Could you check a few things on this model? Use its own coordinates, in mm. Face numbers are marked on the shaded views. A direction names the side the tool comes from. Give positions to 0.01 mm unless a question says otherwise; leave off trailing zeros. Write each loop counter-clockwise with the first axis right and the second up, starting at its lowest first coordinate (ties: lowest second). Pieces come first, ordered by that corner, then holes. Notation, with made-up numbers: M 88,79.5 L 118,79.5 A14 cw 118,97.5 Z; hole C 48.5,-31 d9. An arc over 180 degrees is marked long. Answer as CSV lines item,"result". Start each with the question number.
from build123d import *

# Parameters (mm, degrees)
SKETCH2_R           = 2
BOSS_EXTRUDE1_DEPTH = 11
SKETCH3_R           = 2
BOSS_EXTRUDE2_DEPTH = 39
EXTRUDE_THIN1_REACH = 198.85
CUT_EXTRUDE2_START  = -6
SKETCH5_R           = 3
SKETCH5_R_2         = 2
CUT_EXTRUDE2_DEPTH  = 6


with BuildPart() as part:
    # Sketch2 → Boss-Extrude1 (new body)
    with BuildSketch(Plane(origin=(0, 0, 0), x_dir=(1, 0, 0), z_dir=(0, 1, 0))):
        with BuildLine():
            Line((0, -150), (29.793839815, -175))
            Line((29.793839815, -175), (69, -175))
            ThreePointArc((69, -175), (73.242640687, -173.242640687), (75, -169))
            Line((75, -169), (75, -6))
            ThreePointArc((75, -6), (73.242640687, -1.757359313), (69, 0))
            Line((69, 0), (6, 0))
            ThreePointArc((6, 0), (1.757359313, -1.757359313), (0, -6))
            Line((0, -6), (0, -150))
        make_face()
        with Locations(Location((69, -169, 0), (0, 0, 270))):
            Circle(SKETCH2_R, mode=Mode.SUBTRACT)
        with Locations(Location((69, -6, 0), (0, 0, 270))):
            Circle(SKETCH2_R, mode=Mode.SUBTRACT)
        with Locations(Location((6, -6, 0), (0, 0, 270))):
            Circle(SKETCH2_R, mode=Mode.SUBTRACT)
        with Locations(Location((39, -75, 0), (0, 0, 270))):
            Circle(SKETCH2_R, mode=Mode.SUBTRACT)
    extrude(amount=BOSS_EXTRUDE1_DEPTH)

    # Sketch3 → Boss-Extrude2 (add)
    with BuildSketch(Plane(origin=(0, 11, 0), x_dir=(1, 0, 0), z_dir=(0, 1, 0))):
        with BuildLine():
            Line((39, -67.5), (15, -67.5))
            Line((15, -67.5), (15, -15))
            Line((15, -15), (75, -15))
            Line((75, -15), (75, -6))
            ThreePointArc((75, -6), (73.242640687, -1.757359313), (69, 0))
            Line((69, 0), (6, 0))
            ThreePointArc((6, 0), (1.757359313, -1.757359313), (0, -6))
            Line((0, -6), (0, -150))
            Line((0, -150), (29.793839815, -175))
            Line((29.793839815, -175), (69, -175))
            ThreePointArc((69, -175), (73.242640687, -173.242640687), (75, -169))
            Line((75, -169), (75, -160))
            Line((75, -160), (35.253393329, -160))
            Line((35.253393329, -160), (15, -143.005385128))
            Line((15, -143.005385128), (15, -82.5))
            Line((15, -82.5), (39, -82.5))
            ThreePointArc((39, -82.5), (46.5, -75), (39, -67.5))
        make_face()
        with Locations(Location((69, -169, 0), (0, 0, 270))):
            Circle(SKETCH3_R, mode=Mode.SUBTRACT)
        with Locations(Location((6, -6, 0), (0, 0, 270))):
            Circle(SKETCH3_R, mode=Mode.SUBTRACT)
        with Locations(Location((39, -75, 0), (0, 0, 270))):
            Circle(SKETCH3_R, mode=Mode.SUBTRACT)
        with Locations(Location((69, -6, 0), (0, 0, 270))):
            Circle(SKETCH3_R, mode=Mode.SUBTRACT)
    extrude(amount=BOSS_EXTRUDE2_DEPTH)

    # Sketch4 → Extrude-Thin1 (add, up to next)
    with BuildSketch(Plane(origin=(75, 0, 0), x_dir=(0, 0, -1), z_dir=(1, 0, 0)), mode=Mode.PRIVATE) as extrude_thin1_sk1:
        Polygon((-160, 17.535298339), (-120, 17.535298339), (-100, 11), (-103.106030321, 1.494602815), (-121.592395321, 7.535298339), (-160, 7.535298339), align=None)
    extrude_thin1_tool1 = extrude(extrude_thin1_sk1.sketch, amount=-EXTRUDE_THIN1_REACH, mode=Mode.PRIVATE) - part.part
    add(extrude_thin1_tool1.solids().sort_by_distance((75, 11.508735, 130.439328))[0])

    # Sketch5 → Cut-Extrude2 (cut)
    # profile 1 of 5: a face of its own
    with BuildSketch(Plane(origin=(0, 50, 0), x_dir=(1, 0, 0), z_dir=(0, 1, 0)).offset(CUT_EXTRUDE2_START)):
        with Locations(Location((69, -6, 0), (0, 0, 270))):
            Circle(SKETCH5_R)
        with Locations(Location((69, -6, 0), (0, 0, 270))):
            Circle(SKETCH5_R_2, mode=Mode.SUBTRACT)
    # profile 2 of 5: a face of its own
    with BuildSketch(Plane(origin=(0, 50, 0), x_dir=(1, 0, 0), z_dir=(0, 1, 0)).offset(CUT_EXTRUDE2_START)):
        with Locations(Location((6, -6, 0), (0, 0, 270))):
            Circle(SKETCH5_R)
        with Locations(Location((6, -6, 0), (0, 0, 270))):
            Circle(SKETCH5_R_2, mode=Mode.SUBTRACT)
    # profile 3 of 5: a face of its own
    with BuildSketch(Plane(origin=(0, 50, 0), x_dir=(1, 0, 0), z_dir=(0, 1, 0)).offset(CUT_EXTRUDE2_START)):
        with Locations(Location((39, -75, 0), (0, 0, 270))):
            Circle(SKETCH5_R)
        with Locations(Location((39, -75, 0), (0, 0, 270))):
            Circle(SKETCH5_R_2, mode=Mode.SUBTRACT)
    # profile 4 of 5: a face of its own
    with BuildSketch(Plane(origin=(0, 50, 0), x_dir=(1, 0, 0), z_dir=(0, 1, 0)).offset(CUT_EXTRUDE2_START)):
        with Locations(Location((69, -169, 0), (0, 0, 270))):
            Circle(SKETCH5_R)
        with Locations(Location((69, -169, 0), (0, 0, 270))):
            Circle(SKETCH5_R_2, mode=Mode.SUBTRACT)
    # profile 5 of 5: a face of its own
    with BuildSketch(Plane(origin=(0, 50, 0), x_dir=(1, 0, 0), z_dir=(0, 1, 0)).offset(CUT_EXTRUDE2_START)):
        with Locations(Location((69, -6, 0), (0, 0, 270))):
            Circle(SKETCH5_R_2)
    extrude(amount=CUT_EXTRUDE2_DEPTH, mode=Mode.SUBTRACT)


solid = part.part
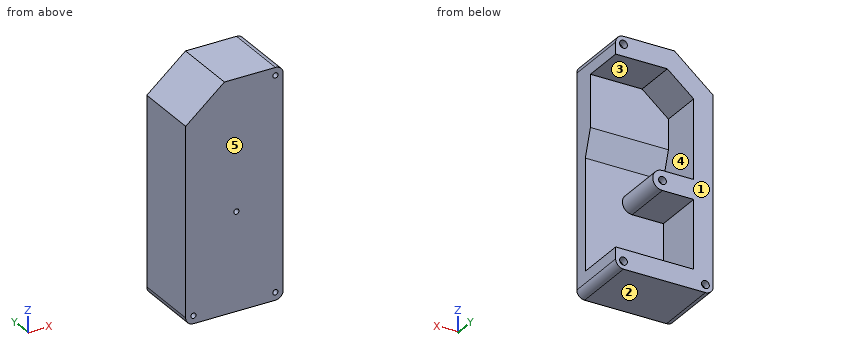
1. Imagine slicing it at A-A, the plane y = 4.5. Please give me the cut outline in (x, z).
2. Imagine slicing it at D-D, the plane y = 23. Please give me the cut outline in (x, z), plus the area to 3 significant figures.
3. Imagine slicing it at C-C, the plane x = 49. Please give me the cut outline in (y, z), plus the area to 3 significant figures.
4. On a 3-axis mill with a long thin cutter (end or side, diameter ignored), from which of +Z, -Z, +X, -X, +Y, -Y can I reach the whole of each face in a straight line? I mean the marked faces 4 and 5. Say none if no direction works.
5. Please list where these lines run through material, in increasing order: line 1 (X direction, y = 46.1, z = 6); line 2 (X direction, y = 14, z = 6); line 3 (X direction, y = 30, z = 75).
6. Imagine slicing it at B-B, the plane z = 75. Please give me the cut outline in (x, y).
7. Will these pins go through, and if not, where does the flat tip stop? P1, Ø1.8, axis at x = 69, z = 7, coming from the +Y side; P2, Ø5.5, axis at x = 39, z = 75, coming from the +Y side; P3, Ø11.5, axis at y = 24, z = 35.5, coming from the +X side; P4, Ø20, axis at x = 51.5, z = 134.5, coming from the +Y side.
8. Thinking about a two-plate mould opening in Z: for the marked faces 1, 2 and 3, which applies, pulls with the +Z half, pulls with the -Z half, needs draft (parallel to the pull), parting line crosses it, or undercut?
Solutions:
1,outline,"M 0,6 A6 ccw 6,0 L 69,0 A6 ccw 75,6 L 75,169 A6 ccw 69,175 L 29.79,175 L 0,150 Z; hole C 6,6 d4; hole C 39,75 d4; hole C 69,6 d4; hole C 69,169 d4"
2,outline,"M 0,6 A6 ccw 6,0 L 69,0 A6 ccw 75,6 L 75,15 L 15,15 L 15,67.5 L 39,67.5 A7.5 ccw 39,82.5 L 15,82.5 L 15,143.01 L 35.25,160 L 75,160 L 75,169 A6 ccw 69,175 L 29.79,175 L 0,150 Z; hole C 6,6 d4; hole C 39,75 d4; hole C 69,6 d4; hole C 69,169 d4"
2,area,"4,600 mm²"
3,outline,"M 0,0 L 50,0 L 50,15 L 11,15 L 11,100 L 17.54,120 L 17.54,160 L 50,160 L 50,175 L 0,175 Z"
3,area,"3,420 mm²"
4,face 4,"+X, +Y"
4,face 5,"+Z, -Z, +X, -X, -Y"
5,line 1,"0 to 3, 9 to 66, 72 to 75"
5,line 2,"0 to 4, 8 to 67, 71 to 75"
5,line 3,"0 to 37, 41 to 46.5"
6,outline,"M 0,0 L 37,0 L 37,44 L 36,44 L 36,50 L 0,50 Z; M 41,0 L 75,0 L 75,11 L 46.5,11 L 46.5,50 L 42,50 L 42,44 L 41,44 Z"
7,P1,"through"
7,P2,"y = 44"
7,P3,"x = 15"
7,P4,"y = 17.54"
8,face 1,"needs draft"
8,face 2,"pulls with the -Z half"
8,face 3,"undercut"
